```python
from build123d import *

# Parameters (mm, degrees)
BOSS_EXTRUDE1_DEPTH      = 14.5
BOSS_EXTRUDE1_DEPTH_BACK = 14.5
SKETCH2_R                = 1.5
CUT_EXTRUDE1_DEPTH       = 14.5


with BuildPart() as part:
    # Sketch1 → Boss-Extrude1 (new, two sides: drawn at the far end of the back side and taken through both)
    with BuildSketch(Plane.XY.offset(-BOSS_EXTRUDE1_DEPTH_BACK)):
        with BuildLine():
            Line((-11.25, -7.125), (-20, -7.125))
            Line((-20, -7.125), (-24, -7.125))
            Line((-24, -7.125), (-24, -4.125))
            Line((-24, -4.125), (-20, -4.125))
            Line((-20, -4.125), (-15.002024714, -4.125))
            ThreePointArc((-15.002024714, -4.125), (-14.270980746, -3.807330358), (-14.004397729, -3.056149435))
            Line((-14.004397729, -3.056149435), (-14.5, 4.125))
            Line((-14.5, 4.125), (-8.746427842, 4.125))
            ThreePointArc((-8.746427842, 4.125), (0, 7.125), (8.746427842, 4.125))
            Line((8.746427842, 4.125), (14.5, 4.125))
            Line((14.5, 4.125), (14.004397729, -3.056149435))
            ThreePointArc((14.004397729, -3.056149435), (14.270980746, -3.807330358), (15.002024714, -4.125))
            Line((15.002024714, -4.125), (20, -4.125))
            Line((20, -4.125), (24, -4.125))
            Line((24, -4.125), (24, -7.125))
            Line((24, -7.125), (20, -7.125))
            Line((20, -7.125), (11.25, -7.125))
            ThreePointArc((11.25, -7.125), (0, 4.125), (-11.25, -7.125))
        make_face()
    extrude(amount=BOSS_EXTRUDE1_DEPTH + BOSS_EXTRUDE1_DEPTH_BACK)

    # Sketch2 → Cut-Extrude1 (cut)
    with BuildSketch(Plane(origin=(0, -4.125, 0), x_dir=(1, 0, 0), z_dir=(0, 1, 0))):
        with Locations(Location((-19.501012357, 0, 0), (0, 0, 270))):
            Circle(SKETCH2_R)
        with Locations(Location((19.501012357, 0, 0), (0, 0, 270))):
            Circle(SKETCH2_R)
    extrude(amount=-CUT_EXTRUDE1_DEPTH, mode=Mode.SUBTRACT)


solid = part.part
```
Source: CAD feature listing. Evaluate the final solid. Frame: model axes, mm. A direction names the side the tool comes from. Round coordinates to 2 decimals unless told otherwise and drop trailing zeros. Loops run counter-clockwise (first coordinate to the right, second up) from the corner with the lowest first, then second, coordinate; pieces in that order, holes last.
(1) Section query D-D (x = 20.5). Output: boundary loops of the cut face in (y, z) (3 decimals).
From the geometry:
outline: (-7.125, -14.5) - (-4.125, -14.5) - (-4.125, -1.119) - (-7.125, -1.119) - close; (-7.125, 1.119) - (-4.125, 1.119) - (-4.125, 14.5) - (-7.125, 14.5) - close
(2) Contact query for flat-ended pins moving along their axis: pin 1 Ø5 at (y, z) = (5.5, -2) entering from -X; pin 2 Ø10 at (x, z) = (-20, 7) entering from +Y (3 decimals); pin 3 Ø1.5 at (y, z) = (0.5, -10.5) entering from -X. Output: stop coordinate, or through.
From the geometry:
pin 1: stops at x = -14.5
pin 2: stops at y = -4.125
pin 3: stops at x = -14.3
(3) Access query for faces 1 (the flat face through (14.256, 0.585, -0.203)), 2 (the cylindrical face through (-14.279, -3.816, -0.203)), 3 (the flat face through (17, -4.125, 0)). Directions: +Z, -Z, +X, -X, +Y, -Y. A direction counts if a zero-diameter tool reaches every point of the face in a straight line with its end or side. Return the directions, or none.
From the geometry:
face 1: +Z, -Z, +X
face 2: +Z, -Z, -X
face 3: +Z, -Z, +X, +Y
(4) Pull-direction query (Y, two-part tool) for faces 4 (the flat face through (-12, 4.125, 0)), 5 (the flat face through (-14.25, 0.48, -0.2)), 6 (the flat face through (24, -6, 0)); classes: +Y half, -Y half, draft (parallel to the pull), parting line (faces both ways), or undercut.
From the geometry:
face 4: +Y half
face 5: undercut
face 6: draft
(5) Section query B-B (y = -5.5). Output: boundary loops of the cut face in (x, z).
From the geometry:
outline: (-24, -14.5) - (-11.13, -14.5) - (-11.13, 14.5) - (-24, 14.5) - close; (11.13, -14.5) - (24, -14.5) - (24, 14.5) - (11.13, 14.5) - close; hole circle Ø3 at (-19.5, 0); hole circle Ø3 at (19.5, 0)
(6) Section query C-C (z = 7.25). Output: boundary loops of the cut face in (x, y) (3 decimals), and give its area (3 significant figures).
From the geometry:
outline: (-24, -7.125) - (-11.25, -7.125) arc R11.25 cw to (11.25, -7.125) - (24, -7.125) - (24, -4.125) - (15.002, -4.125) arc R1 cw to (14.004, -3.056) - (14.5, 4.125) - (8.746, 4.125) arc R14.25 ccw to (-8.746, 4.125) - (-14.5, 4.125) - (-14.004, -3.056) arc R1 cw to (-15.002, -4.125) - (-24, -4.125) - close
area: 216 mm2
(7) Section query A-A (z = 0). Output: boundary loops of the cut face in (x, y) (3 decimals).
From the geometry:
outline: (-24, -7.125) - (-21.001, -7.125) - (-21.001, -4.125) - (-24, -4.125) - close; (-18.001, -7.125) - (-11.25, -7.125) arc R11.25 cw to (11.25, -7.125) - (18.001, -7.125) - (18.001, -4.125) - (15.002, -4.125) arc R1 cw to (14.004, -3.056) - (14.5, 4.125) - (8.746, 4.125) arc R14.25 ccw to (-8.746, 4.125) - (-14.5, 4.125) - (-14.004, -3.056) arc R1 cw to (-15.002, -4.125) - (-18.001, -4.125) - close; (21.001, -7.125) - (24, -7.125) - (24, -4.125) - (21.001, -4.125) - close
(8) Material intervals for probe 1 along X at (y, z) = (-4.65, 0); probe 2 along X at (y, z) = (-5.95, 0); probe 3 along X at (y, z) = (-4, 3), sorted ascending.
From the geometry:
probe 1: x = -24 to -21, -18 to -10.97, 10.97 to 18, 21 to 24
probe 2: x = -24 to -21, -18 to -11.19, 11.19 to 18, 21 to 24
probe 3: x = -14.52 to -10.81, 10.81 to 14.52
